```python
from build123d import *

# Parameters (mm, degrees)
SKETCH1_W                    = 40
SKETCH1_H                    = 15
BASE_FLANGE1_DEPTH           = 0.5
EDGE_FLANGE1_STRIP_W         = 3
EDGE_FLANGE1_STRIP_H         = 0.5
EDGE_FLANGE1_STRIP_CUT_DEPTH = 40
EDGE_FLANGE1_DEPTH           = 40
F_6_CLEARANCE_HOLE2_D        = 3.7973
F_6_CLEARANCE_HOLE2_DEPTH    = 10
F_6_CLEARANCE_HOLE2_TIP      = 1.140824014
F_6_CLEARANCE_HOLE3_D        = 3.7973
BREAK_CORNER1_START          = -10
BREAK_CORNER1_DEPTH          = 0.5
BREAK_CORNER1_START_2        = -0.5
BREAK_CORNER1_2_DEPTH        = 0.5


# Read off the part's stored shape, not the designer's step: Break-Corner1
# Sheet-metal steps are written as plain solids
with BuildPart() as part:
    # Sketch1 → Base-Flange1 (new body)
    with BuildSketch(Plane(origin=(0, 0, 0), x_dir=(1, 0, 0), z_dir=(0, 1, 0))):
        with Locations((0, 2.5)):
            Rectangle(SKETCH1_W, SKETCH1_H)
    extrude(amount=-BASE_FLANGE1_DEPTH)

    # Edge-Flange1 strip (across the edge) → Edge-Flange1 strip cut (cut)
    with BuildSketch(Plane(origin=(-20, -0.5, -10), x_dir=(0, 0, 1), z_dir=(1, 0, 0))):
        with Locations((-0.5, -0.25)):
            Rectangle(EDGE_FLANGE1_STRIP_W, EDGE_FLANGE1_STRIP_H)
    extrude(amount=EDGE_FLANGE1_STRIP_CUT_DEPTH, mode=Mode.SUBTRACT)

    # Edge-Flange1 section (across the edge) → Edge-Flange1 (add)
    with BuildSketch(Plane(origin=(-20, -0.5, -10), x_dir=(0, 0, 1), z_dir=(1, 0, 0))):
        with BuildLine():
            Line((0, 0.5), (0, 14.5))
            Line((0, 14.5), (0.5, 14.5))
            Line((0.5, 14.5), (0.5, 0.5))
            ThreePointArc((0.5, 0.5), (0.646446609, 0.146446609), (1, 0))
            Line((1, 0), (1, -0.5))
            ThreePointArc((1, -0.5), (0.292893219, -0.207106781), (0, 0.5))
        make_face()
    extrude(amount=EDGE_FLANGE1_DEPTH)

    # #6 Clearance Hole2
    with Locations(Plane.XY.offset(-9.5)):
        with Locations((-9, -6), (9, -6)):
            Hole(F_6_CLEARANCE_HOLE2_D / 2, depth=F_6_CLEARANCE_HOLE2_DEPTH)
            with Locations((0, 0, -(F_6_CLEARANCE_HOLE2_DEPTH + F_6_CLEARANCE_HOLE2_TIP / 2))):  # 118° drill point
                Cone(0, F_6_CLEARANCE_HOLE2_D / 2, F_6_CLEARANCE_HOLE2_TIP, mode=Mode.SUBTRACT)

    # #6 Clearance Hole3 (through all)
    with Locations(Plane(origin=(0, 0, 0), x_dir=(1, 0, 0), z_dir=(0, 1, 0))):
        with Locations((12, 4), (-12, 4)):
            Hole(F_6_CLEARANCE_HOLE3_D / 2)

    # Break-Corner1 outline → Break-Corner1 (cut)
    with BuildSketch(Plane.XY.offset(BREAK_CORNER1_START)):
        with BuildLine():
            Line((-20, -15), (-15, -15))
            ThreePointArc((-15, -15), (-18.535533906, -13.535533906), (-20, -10))
            Line((-20, -10), (-20, -15))
        make_face()
        with BuildLine():
            ThreePointArc((20, -10), (18.535533906, -13.535533906), (15, -15))
            Line((15, -15), (20, -15))
            Line((20, -15), (20, -10))
        make_face()
    extrude(amount=BREAK_CORNER1_DEPTH, mode=Mode.SUBTRACT)

    # Break-Corner1 2 outline → Break-Corner1 2 (cut)
    with BuildSketch(Plane(origin=(0, 0, 0), x_dir=(1, 0, 0), z_dir=(0, 1, 0)).offset(BREAK_CORNER1_START_2)):
        with BuildLine():
            ThreePointArc((20, 0), (18.535533906, -3.535533906), (15, -5))
            Line((15, -5), (20, -5))
            Line((20, -5), (20, 0))
        make_face()
        with BuildLine():
            ThreePointArc((-15, -5), (-18.535533906, -3.535533906), (-20, 0))
            Line((-20, 0), (-20, -5))
            Line((-20, -5), (-15, -5))
        make_face()
    extrude(amount=BREAK_CORNER1_2_DEPTH, mode=Mode.SUBTRACT)


solid = part.part
```
For this review, take the finished solid that the model builds, in its own axes (mm). A direction names the side the tool comes from. Coordinates: 2 decimals unless noted, no trailing zeros. Loops run counter-clockwise (first coordinate to the right, second up) from the corner with the lowest first, then second, coordinate; pieces in that order, holes last.
1. Insertion check: P1, Ø1.5, axis at x = 1, z = 3.5, coming from the -Y side; P2, Ø6, axis at x = -2.5, y = -2.5, coming from the +Z side; P3, Ø8, axis at x = -12.5, y = -11, coming from the +Z side. Each pin has a flat end and moves straight along its axis. Give the tip position at first contact, or say it passes through.
2. For faces 1 (the flat face through (0, -0.5, -2)), 2 (the cylindrical face through (18.57, -13.5, -9.75)), list the 3-axis set-ups (+Z, -Z, +X, -X, +Y, -Y) from which the entire face can be reached by the end or side of a thin tool; tool diameter is ignored.
3. Add section B-B, the plane z = -4. Give the boundary of the cut face in (x, y), then the cut area to 3 significant figures.
4. Add section A-A, the plane y = -6. Give the boundary of the cut face in (x, z), then the cut area to 3 significant figures.
5. Add section C-C, the plane x = -9. Give the boundary of the cut face in (y, z), then the cut area to 3 significant figures.
6. Add section D-D, the plane y = -3. Give the boundary of the cut face in (x, z), then the cut area to 3 significant figures.
7. For line 1 (Z direction, x = 2, y = -6.75); line 2 (Y direction, x = -16, z = -3.75); line 3 (Y direction, x = -9, z = -9.65), list the stretches that pass through material, from the lowest coordinate up.
8. Mouldability with a two-part tool opening along Z and no side actions: class faces 3 (the flat face through (0, -8, -9.5)), 4 (the cylindrical face through (13.897, -0.254, -4.083)), 5 (the flat face through (0, -8, -10)), 6 (the flat face through (-20, -0.2, -7.2)) as +Z half, -Z half, draft (parallel to the pull), parting line (faces both ways), or undercut.
Result:
1. P1: stops at y = -0.5
1. P2: stops at z = 5
1. P3: stops at z = -9.5
2. face 1: +Z, +X, -X, -Y
2. face 2: +Z, -Z, +X, -Y
3. outline: (-20, -0.5) - (-13.9, -0.5) - (-13.9, 0) - (-20, 0) - close; (-10.1, -0.5) - (10.1, -0.5) - (10.1, 0) - (-10.1, 0) - close; (13.9, -0.5) - (20, -0.5) - (20, 0) - (13.9, 0) - close
3. area: 16.2 mm2
4. outline: (-20, -10) - (-10.9, -10) - (-10.9, -9.5) - (-20, -9.5) - close; (-7.1, -10) - (7.1, -10) - (7.1, -9.5) - (-7.1, -9.5) - close; (10.9, -10) - (20, -10) - (20, -9.5) - (10.9, -9.5) - close
4. area: 16.2 mm2
5. outline: (-15, -10) - (-7.9, -10) - (-7.9, -9.5) - (-15, -9.5) - close; (-4.1, -10) - (-1, -10) arc R1 ccw to (0, -9) - (0, 5) - (-0.5, 5) - (-0.5, -9) arc R0.5 cw to (-1, -9.5) - (-4.1, -9.5) - close
5. area: 12.7 mm2
6. outline: (-20, -10) - (20, -10) - (20, -9.5) - (-20, -9.5) - close
6. area: 20.0 mm2
7. line 1: z = -10 to -9.5
7. line 2: y = -0.5 to 0
7. line 3: y = -15 to -7.9, -4.1 to -0.24
8. face 3: +Z half
8. face 4: undercut
8. face 5: -Z half
8. face 6: draft
